from build123d import *

# Parameters (mm, degrees)
F2_DEPTH = 17.5
F3_W     = 12.5
F3_H     = 25


with BuildPart() as f1:
    # F0 (on Front) → F1 (revolve)
    with BuildSketch(Plane.XZ):
        Polygon((0, 20), (0, 0), (37.5, 0), (37.5, 20), (17.5, 20), align=None)
    revolve(axis=Axis((0, 0, 47), (0, 0, -1)))

    # F0 (on Front) → F2 (join, symmetric)
    with BuildSketch(Plane.XZ):
        Polygon((0, 57), (0, 20), (17.5, 20), (17.5, 57), (12.5, 57), align=None)
    extrude(amount=F2_DEPTH, both=True)

    # F3 (on face) → F6 section 0
    with BuildSketch(Plane.XY.offset(57), mode=Mode.PRIVATE) as f6_s0:
        with Locations((6.25, 0)):
            Rectangle(F3_W, F3_H)
    loft([f6_s0.sketch, Vertex(0, 0, 94)])

    # F7: F1 across plane


with BuildPart() as f1_1:
    add(f1.part)
    add(f1.part.mirror(Plane.YZ))


solid = f1_1.part
The model under review builds one solid part; all positions refer to its coordinate system, in mm. A direction names the side the tool comes from. Round coordinates to 2 decimals unless told otherwise and drop trailing zeros. Loops run counter-clockwise (first coordinate to the right, second up) from the corner with the lowest first, then second, coordinate; pieces in that order, holes last. Notation, with made-up numbers: M 61.25,81 L 104.25,81 A12 cw 104.25,89 Z; hole C 17,83.25 d4. An arc over 180 degrees is marked long. Answer as CSV lines item,"result". Start each with the question number.
Item 1: Consider section B-B (z = 27). Write out the cut boundary in (x, y), then the cut area to 4 significant figures.
Item 2: Consider section C-C (y = 15). Write out the cut boundary in (x, z), then the cut area to 3 significant figures.
Item 3: Consider section A-A (x = -7). Write out the cut boundary in (y, z), then the cut area to 3 significant figures.
Item 4: For faces 1 (the face through (17.5, 0, 38)), 2 (the face through (16, 0, 57)), 3 (the face through (0, -17.5, 39)), 4 (the face through (0, 17.5, 39)), list the 3-axis set-ups (+Z, -Z, +X, -X, +Y, -Y) from which the entire face can be reached by the end or side of a thin tool; tool diameter is ignored.
Item 5: Wall thickness on line 1 (Y direction, x = 7.5, z = 36); line 2 (Z direction, x = 14, y = 17); line 3 (Z direction, x = 9, y = -22): over which ranges is each line inside the solid? List them lowest first. Write a range as [from, to].
Item 6: Insertion check: P1, Ø1, axis at x = -13.5, y = -11, coming from the +Z side; P2, Ø10.5, axis at x = -1, z = 42, coming from the +Y side; P3, Ø12, axis at x = -2, z = 79.5, coming from the +Y side. Each pin has a flat end and moves straight along its axis. Give the tip position at first contact, or say it passes through.
Item 7: Consider section D-D (y = 27). Write out the cut boundary in (x, z).
Answer:
1,outline,"M -17.5,-17.5 L 17.5,-17.5 L 17.5,17.5 L -17.5,17.5 Z"
1,area,"1,225 mm^2"
2,outline,"M -34.37,0 L 34.37,0 L 34.37,20 L 17.5,20 L 17.5,57 L -17.5,57 L -17.5,20 L -34.37,20 Z"
2,area,"2,670 mm^2"
3,outline,"M -36.84,0 L 36.84,0 L 36.84,20 L 17.5,20 L 17.5,57 L 12.5,57 L 7,73.28 L -7,73.28 L -12.5,57 L -17.5,57 L -17.5,20 L -36.84,20 Z"
3,area,"3,090 mm^2"
4,face 1,"+Z, +X, +Y, -Y"
4,face 2,"+Z"
4,face 3,"+Z, +X, -X, -Y"
4,face 4,"+Z, +X, -X, +Y"
5,line 1,"y = [-17.5, 17.5]"
5,line 2,"z = [0, 57]"
5,line 3,"z = [0, 20]"
6,P1,"stops at z = 57"
6,P2,"stops at y = 17.5"
6,P3,"stops at y = 6.93"
7,outline,"M -26.02,0 L 26.02,0 L 26.02,20 L -26.02,20 Z"
